Design review of the part built by this model. Coordinates are the model's own, in mm. A direction names the side the tool comes from. Coordinates: 2 decimals unless noted, no trailing zeros. Loops run counter-clockwise (first coordinate to the right, second up) from the corner with the lowest first, then second, coordinate; pieces in that order, holes last. Notation, with made-up numbers: M 73.25,16.5 L 114.25,16.5 A6 cw 114.25,27.5 Z; hole C 70,76.5 d2. An arc over 180 degrees is marked long. Answer as a JSON object with one key per item and string values. Group by question number.
1. Insertion check: pin 1 (8 mm diameter, centred on x = 32.5, z = -107.5, fed in from +Y). The pin has a flat end and moves straight along its axis. Give the tip position at first contact, or say it passes through.
2. Consider section B-B (z = -43). State the section outline as (x, y) points.
3. Consider section C-C (x = 73). State the section outline as (y, z) points, then the cut area to 3 significant figures.
4. Machinability: for faces 5 (the flat face through (141.086, -4.24, -99.469)), 6 (the flat face through (161, -3.5, -58)), 7 (the flat face through (-5, 13, -57)), which of the approach directions +Z, -Z, +X, -X, +Y, -Y give a long, thin tool a straight path to every point of the face, cutting with its end or side? Answer none if there is none.
5. Consider section D-D (x = 10). State the section outline as (y, z) points.
6. Draft analysis for pull direction Z (two halves, no side actions). For faces 1 (the flat face through (144, -3.5, -29)), 2 (the flat face through (209.14, 13, -59)), 3 (the flat face through (101, 13, -121)), 4 (the flat face through (72.886, -4.24, -99.469)), state which applies: +Z half, -Z half, draft (parallel to the pull), parting line (faces both ways), or undercut.
7. To check wall thickness, follow probe 1 along X at (y, z) = (4, -61.5); probe 2 along Z at (x, y) = (152.5, 13); probe 3 along Y at (x, z) = (169, -18.5). State the ranges of each line that lie inside material, in increasing order.
8. Consider section A-A (y = 24.5). State the section outline as (x, z) points.
from build123d import *

# Parameters (mm, degrees)
SKETCH1_W           = 14.1
SKETCH1_H           = 14.1
BOSS_EXTRUDE1_DEPTH = 5
BOSS_EXTRUDE2_START = 30
SKETCH1_3_W         = 204.140411229
SKETCH1_3_H         = 116
SKETCH1_3_W_2       = 14.1
SKETCH1_3_H_2       = 14.1
SKETCH1_3_R         = 4.175
SKETCH1_3_W_3       = 10.8
SKETCH1_3_H_3       = 2.5
BOSS_EXTRUDE2_DEPTH = 30
SKETCH3_W           = 18.1
SKETCH3_H           = 18.1
CUT_EXTRUDE1_DEPTH  = 3.5
SKETCH4_W           = 15
SKETCH4_H           = 15
CUT_EXTRUDE2_DEPTH  = 3


with BuildPart() as part:
    # Sketch1 → Boss-Extrude1 (new body)
    with BuildSketch(Plane(origin=(0, 0, 0), x_dir=(1, 0, 0), z_dir=(0, 1, 0))):
        with BuildLine():
            Line((-5, 116), (-5, 0))
            ThreePointArc((-5, 0), (-3.535533906, -3.535533906), (0, -5))
            Line((0, -5), (204.140411229, -5))
            ThreePointArc((204.140411229, -5), (207.675945135, -3.535533906), (209.140411229, 0))
            Line((209.140411229, 0), (209.140411229, 116))
            ThreePointArc((209.140411229, 116), (207.675945135, 119.535533906), (204.140411229, 121))
            Line((204.140411229, 121), (0, 121))
            ThreePointArc((0, 121), (-3.535533906, 119.535533906), (-5, 116))
        make_face()
        with Locations((50.920205615, 58)):
            Rectangle(SKETCH1_W, SKETCH1_H, mode=Mode.SUBTRACT)
        with Locations((85.020205615, 58)):
            Rectangle(SKETCH1_W, SKETCH1_H, mode=Mode.SUBTRACT)
        with Locations((67.970205615, 28.9)):
            Rectangle(SKETCH1_W, SKETCH1_H, mode=Mode.SUBTRACT)
        with Locations((136.170205615, 28.9)):
            Rectangle(SKETCH1_W, SKETCH1_H, mode=Mode.SUBTRACT)
        with Locations((119.120205615, 58)):
            Rectangle(SKETCH1_W, SKETCH1_H, mode=Mode.SUBTRACT)
        with Locations((153.220205615, 58)):
            Rectangle(SKETCH1_W, SKETCH1_H, mode=Mode.SUBTRACT)
        Polygon((77.940411229, 94.414213562), (67.970205615, 84.444007948), (58, 94.414213562), (67.970205615, 104.384419177), align=None, mode=Mode.SUBTRACT)
        Polygon((126.2, 94.414213562), (136.170205615, 104.384419177), (146.140411229, 94.414213562), (136.170205615, 84.444007948), align=None, mode=Mode.SUBTRACT)
        with BuildLine():
            Line((16.185786438, 93.164213562), (16.185786438, 95.664213562))
            Line((16.185786438, 95.664213562), (17.60230492, 95.664213562))
            ThreePointArc((17.60230492, 95.664213562), (21.585786438, 98.589213562), (25.569267955, 95.664213562))
            Line((25.569267955, 95.664213562), (26.985786438, 95.664213562))
            Line((26.985786438, 95.664213562), (26.985786438, 93.164213562))
            Line((26.985786438, 93.164213562), (25.569267955, 93.164213562))
            ThreePointArc((25.569267955, 93.164213562), (21.585786438, 90.239213562), (17.60230492, 93.164213562))
            Line((17.60230492, 93.164213562), (16.185786438, 93.164213562))
        make_face(mode=Mode.SUBTRACT)
        with BuildLine():
            Line((177.154624792, 93.164213562), (177.154624792, 95.664213562))
            Line((177.154624792, 95.664213562), (178.571143274, 95.664213562))
            ThreePointArc((178.571143274, 95.664213562), (182.554624792, 98.589213562), (186.538106309, 95.664213562))
            Line((186.538106309, 95.664213562), (187.954624792, 95.664213562))
            Line((187.954624792, 95.664213562), (187.954624792, 93.164213562))
            Line((187.954624792, 93.164213562), (186.538106309, 93.164213562))
            ThreePointArc((186.538106309, 93.164213562), (182.554624792, 90.239213562), (178.571143274, 93.164213562))
            Line((178.571143274, 93.164213562), (177.154624792, 93.164213562))
        make_face(mode=Mode.SUBTRACT)
    extrude(amount=-BOSS_EXTRUDE1_DEPTH)

    # Sketch1<3> → Boss-Extrude2 (add)
    # profile 1 of 13: a face of its own
    with BuildSketch(Plane(origin=(0, 0, 0), x_dir=(1, 0, 0), z_dir=(0, 1, 0)).offset(BOSS_EXTRUDE2_START)):
        with BuildLine():
            Line((-5, 0), (-5, 116))
            ThreePointArc((-5, 116), (-3.535533906, 119.535533906), (0, 121))
            Line((0, 121), (204.140411229, 121))
            ThreePointArc((204.140411229, 121), (207.675945135, 119.535533906), (209.140411229, 116))
            Line((209.140411229, 116), (209.140411229, 0))
            ThreePointArc((209.140411229, 0), (207.675945135, -3.535533906), (204.140411229, -5))
            Line((204.140411229, -5), (0, -5))
            ThreePointArc((0, -5), (-3.535533906, -3.535533906), (-5, 0))
        make_face()
        with Locations((102.070205615, 58)):
            Rectangle(SKETCH1_3_W, SKETCH1_3_H, mode=Mode.SUBTRACT)
    # profile 2 of 13: a face of its own
    with BuildSketch(Plane(origin=(0, 0, 0), x_dir=(1, 0, 0), z_dir=(0, 1, 0)).offset(BOSS_EXTRUDE2_START)):
        Polygon((136.170205615, 84.444007948), (126.2, 94.414213562), (136.170205615, 104.384419177), (146.140411229, 94.414213562), align=None)
    # profile 3 of 13: a face of its own
    with BuildSketch(Plane(origin=(0, 0, 0), x_dir=(1, 0, 0), z_dir=(0, 1, 0)).offset(BOSS_EXTRUDE2_START)):
        Polygon((67.970205615, 104.384419177), (58, 94.414213562), (67.970205615, 84.444007948), (77.940411229, 94.414213562), align=None)
    # profile 4 of 13: a face of its own
    with BuildSketch(Plane(origin=(0, 0, 0), x_dir=(1, 0, 0), z_dir=(0, 1, 0)).offset(BOSS_EXTRUDE2_START)):
        with Locations((153.220205615, 58)):
            Rectangle(SKETCH1_3_W_2, SKETCH1_3_H_2)
    # profile 5 of 13: a face of its own
    with BuildSketch(Plane(origin=(0, 0, 0), x_dir=(1, 0, 0), z_dir=(0, 1, 0)).offset(BOSS_EXTRUDE2_START)):
        with Locations((119.120205615, 58)):
            Rectangle(SKETCH1_3_W_2, SKETCH1_3_H_2)
    # profile 6 of 13: a face of its own
    with BuildSketch(Plane(origin=(0, 0, 0), x_dir=(1, 0, 0), z_dir=(0, 1, 0)).offset(BOSS_EXTRUDE2_START)):
        with Locations((136.170205615, 28.9)):
            Rectangle(SKETCH1_3_W_2, SKETCH1_3_H_2)
    # profile 7 of 13: a face of its own
    with BuildSketch(Plane(origin=(0, 0, 0), x_dir=(1, 0, 0), z_dir=(0, 1, 0)).offset(BOSS_EXTRUDE2_START)):
        with Locations((67.970205615, 28.9)):
            Rectangle(SKETCH1_3_W_2, SKETCH1_3_H_2)
    # profile 8 of 13: a face of its own
    with BuildSketch(Plane(origin=(0, 0, 0), x_dir=(1, 0, 0), z_dir=(0, 1, 0)).offset(BOSS_EXTRUDE2_START)):
        with Locations((85.020205615, 58)):
            Rectangle(SKETCH1_3_W_2, SKETCH1_3_H_2)
    # profile 9 of 13: a face of its own
    with BuildSketch(Plane(origin=(0, 0, 0), x_dir=(1, 0, 0), z_dir=(0, 1, 0)).offset(BOSS_EXTRUDE2_START)):
        with Locations((50.920205615, 58)):
            Rectangle(SKETCH1_3_W_2, SKETCH1_3_H_2)
    # profile 10 of 13: a face of its own
    with BuildSketch(Plane(origin=(0, 0, 0), x_dir=(1, 0, 0), z_dir=(0, 1, 0)).offset(BOSS_EXTRUDE2_START)):
        with Locations((182.554624792, 94.414213562)):
            Circle(SKETCH1_3_R)
    # profile 11 of 13: a face of its own
    with BuildSketch(Plane(origin=(0, 0, 0), x_dir=(1, 0, 0), z_dir=(0, 1, 0)).offset(BOSS_EXTRUDE2_START)):
        with Locations((21.585786438, 94.414213562)):
            Circle(SKETCH1_3_R)
    # profile 12 of 13: a face of its own
    with BuildSketch(Plane(origin=(0, 0, 0), x_dir=(1, 0, 0), z_dir=(0, 1, 0)).offset(BOSS_EXTRUDE2_START)):
        with Locations((21.585786438, 94.414213562)):
            Rectangle(SKETCH1_3_W_3, SKETCH1_3_H_3)
    # profile 13 of 13: a face of its own
    with BuildSketch(Plane(origin=(0, 0, 0), x_dir=(1, 0, 0), z_dir=(0, 1, 0)).offset(BOSS_EXTRUDE2_START)):
        with Locations((182.554624792, 94.414213562)):
            Rectangle(SKETCH1_3_W_3, SKETCH1_3_H_3)
    extrude(amount=-BOSS_EXTRUDE2_DEPTH)


with BuildPart() as boss_extrude2_kept_piece:
    # of the separate pieces the step leaves, the one the design keeps (boss_extrude2_pieces_kept)
    add(part.part.solids().sort_by_distance((204.140411229, -5, -121))[0])

    # Sketch3 → Cut-Extrude1 (cut)
    with BuildSketch(Plane(origin=(0, 0, 0), x_dir=(1, 0, 0), z_dir=(0, 1, 0))):
        with Locations((50.920205615, 58)):
            Rectangle(SKETCH3_W, SKETCH3_H)
        Polygon((67.970205615, 107.212846302), (55.171572875, 94.414213562), (67.970205615, 81.615580823), (80.768838354, 94.414213562), align=None)
        with Locations((67.970205615, 28.9)):
            Rectangle(SKETCH3_W, SKETCH3_H)
        with Locations((85.020205615, 58)):
            Rectangle(SKETCH3_W, SKETCH3_H)
        with Locations((119.120205615, 58)):
            Rectangle(SKETCH3_W, SKETCH3_H)
        with Locations((153.220205615, 58)):
            Rectangle(SKETCH3_W, SKETCH3_H)
        Polygon((123.371572875, 94.414213562), (136.170205615, 81.615580823), (148.968838354, 94.414213562), (136.170205615, 107.212846302), align=None)
        with Locations((136.170205615, 28.9)):
            Rectangle(SKETCH3_W, SKETCH3_H)
    extrude(amount=-CUT_EXTRUDE1_DEPTH, mode=Mode.SUBTRACT)

    # Sketch4 → Cut-Extrude2 (cut)
    with BuildSketch(Plane(origin=(0, 0, 0), x_dir=(1, 0, 0), z_dir=(0, 1, 0))):
        with Locations((21.585786438, 94.414213562)):
            Rectangle(SKETCH4_W, SKETCH4_H)
        with Locations((182.554624792, 94.414213562)):
            Rectangle(SKETCH4_W, SKETCH4_H)
    extrude(amount=-CUT_EXTRUDE2_DEPTH, mode=Mode.SUBTRACT)


solid = boss_extrude2_kept_piece.part
Findings below:
{
 "1": {"pin 1": "stops at y = 0"},
 "2": {"outline": "M -5,-5 L 209.14,-5 L 209.14,30 L 204.14,30 L 204.14,0 L 0,0 L 0,30 L -5,30 Z"},
 "3": {"outline": "M -5,-121 L 30,-121 L 30,-116 L 0,-116 L 0,-102.18 L -3.5,-102.18 L -3.5,-99.35 L -5,-99.35 Z; M -5,-89.47 L -3.5,-89.47 L -3.5,-86.65 L 0,-86.65 L 0,-37.95 L -3.5,-37.95 L -3.5,-35.95 L -5,-35.95 Z; M -5,-21.85 L -3.5,-21.85 L -3.5,-19.85 L 0,-19.85 L 0,0 L 30,0 L 30,5 L -5,5 Z", "area": "776 mm^2"},
 "4": {"face 5": "+Y, -Y", "face 6": "+Y", "face 7": "+Z, -Z, -X, +Y, -Y"},
 "5": {"outline": "M -5,-121 L 30,-121 L 30,-116 L 0,-116 L 0,0 L 30,0 L 30,5 L -5,5 Z"},
 "6": {"face 1": "undercut", "face 2": "draft", "face 3": "-Z half", "face 4": "undercut"},
 "7": {"probe 1": "x = -5 to 0, 204.14 to 209.14", "probe 2": "z = -121 to -116, 0 to 5", "probe 3": "y = -5 to 0"},
 "8": {"outline": "M -5,-116 A5 ccw 0,-121 L 204.14,-121 A5 ccw 209.14,-116 L 209.14,0 A5 ccw 204.14,5 L 0,5 A5 ccw -5,0 Z; hole M 0,-116 L 204.14,-116 L 204.14,0 L 0,0 Z"}
}
